from build123d import *

# Parameters (mm, degrees)
SKETCH_1_W               = 56
SKETCH_1_H               = 40
EXTRUDE_1_DEPTH          = 20
SKETCH_2_R               = 7.5
CUT_EXTRUDE_1_DEPTH      = 48
CUT_EXTRUDE_2_DEPTH      = 70.503098378
CUT_EXTRUDE_2_DEPTH_BACK = 48
SKETCH_5_R               = 4.15
CUT_EXTRUDE_3_DEPTH      = 10
SKETCH_6_R               = 2.1
CUT_EXTRUDE_4_DEPTH      = 57.255246128
CUT_EXTRUDE_5_DEPTH      = 10


with BuildPart() as part:
    # Эскиз1 → Бобышка-Вытянуть1 (new body)
    with BuildSketch(Plane(origin=(0, 0, 0), x_dir=(1, 0, 0), z_dir=(0, 1, 0))):
        with Locations((-4.217573352, -21.553347449)):
            Rectangle(SKETCH_1_W, SKETCH_1_H)
    extrude(amount=EXTRUDE_1_DEPTH)

    # Эскиз2 → Вырез-Вытянуть1 (cut)
    with BuildSketch(Plane.ZY.offset(28.217573352)):
        with Locations((39.13573239, 10)):
            Circle(SKETCH_2_R)
    extrude(amount=-CUT_EXTRUDE_1_DEPTH, mode=Mode.SUBTRACT)

    # Эскиз4 → Вырез-Вытянуть2 (cut, two sides: drawn at the far end of the back side and taken through both)
    with BuildSketch(Plane.ZY.offset(-19.782426648).offset(-CUT_EXTRUDE_2_DEPTH_BACK)):
        with BuildLine():
            Line((37.693734465, 13.535), (41.553347449, 13.535))
            Line((41.553347449, 13.535), (41.553347449, 6.465))
            Line((41.553347449, 6.465), (37.693734465, 6.465))
            ThreePointArc((37.693734465, 6.465), (34.158734465, 10), (37.693734465, 13.535))
        make_face()
    extrude(amount=CUT_EXTRUDE_2_DEPTH + CUT_EXTRUDE_2_DEPTH_BACK, mode=Mode.SUBTRACT)

    # Эскиз5 → Вырез-Вытянуть3 (cut)
    with BuildSketch(Plane(origin=(0, 0, 1.553347449), x_dir=(-1, 0, 0), z_dir=(0, 0, -1))):
        with Locations((-16.782426648, 10)):
            Circle(SKETCH_5_R)
        with Locations((25.217573352, 10)):
            Circle(SKETCH_5_R)
    extrude(amount=-CUT_EXTRUDE_3_DEPTH, mode=Mode.SUBTRACT)

    # Эскиз6 → Вырез-Вытянуть4 (cut, through all)
    with BuildSketch(Plane(origin=(0, 20, 0), x_dir=(1, 0, 0), z_dir=(0, 1, 0))):
        with Locations(Location((-25.217573352, -21.553347449, 0), (0, 0, 270))):
            Circle(SKETCH_6_R)
        with Locations(Location((16.782426648, -21.553347449, 0), (0, 0, 270))):
            Circle(SKETCH_6_R)
    extrude(amount=-CUT_EXTRUDE_4_DEPTH, mode=Mode.SUBTRACT)

    # Эскиз7 → Вырез-Вытянуть5 (cut)
    with BuildSketch(Plane.XZ):
        Polygon((-21.176121468, 21.553347449), (-23.19684741, 25.053347449), (-27.238299295, 25.053347449), (-29.259025237, 21.553347449), (-27.238299295, 18.053347449), (-23.19684741, 18.053347449), align=None)
        Polygon((20.823878532, 21.553347449), (18.80315259, 25.053347449), (14.761700705, 25.053347449), (12.740974763, 21.553347449), (14.761700705, 18.053347449), (18.80315259, 18.053347449), align=None)
    extrude(amount=-CUT_EXTRUDE_5_DEPTH, mode=Mode.SUBTRACT)


solid = part.part
Work out the finished part from the listing and answer in its coordinate system (mm). A direction names the side the tool comes from. Round coordinates to 2 decimals unless told otherwise and drop trailing zeros. Write each loop counter-clockwise with the first axis right and the second up, starting at its lowest first coordinate (ties: lowest second). Pieces come first, ordered by that corner, then holes.
1) Given pin 1 Ø1.2 at (x, z) = (21, 38.5) entering from -Y; pin 2 Ø2 at (x, z) = (-27, 20) entering from -Y; pin 3 Ø8 at (x, y) = (1, 12.5) entering from +Z; pin 4 Ø4 at (x, y) = (15.5, 10.5) entering from -Z, each flat-ended and moving along its own axis, determine where each tip first touches the part or whether it passes through.
2) A tool of negligible diameter and unlimited length cuts with its end or side. For faces 4 (the cylindrical face through (-4.55, 10.2, 31.64)), 5 (the flat face through (13.765, 4.93, 23.328)), 6 (the flat face through (-30, 6.465, 40)), from which of +Z, -Z, +X, -X, +Y, -Y can it reach the whole face along a straight path? Write none if from no direction.
3) Straight lines are drawn through the part: line 1 (X direction, y = 8.5, z = 6); line 2 (Y direction, x = -19, z = 38); line 3 (Y direction, x = 8, z = 35.5). For each, find the intervals that lie inside material, in ascending order.
4) The mould has two halves that part along Z. Classify faces 1 (the flat face through (22, 6.465, 40)), 2 (the flat face through (19.8, 4.93, 19.78)), 3 (the cylindrical face through (-30.19, 9.92, 34.16)): pulls with the +Z half, pulls with the -Z half, needs draft (parallel to the pull), parting line crosses it, or undercut.
5) A cutting plane is placed at B-B (x = -24). Give the vertices of the cut face in (y, z), plus the area to 3 significant figures.
6) A cutting plane is placed at C-C (x = 4). Give the vertices of the cut face in (y, z).
7) A cutting plane is placed at A-A (z = 8). Give the vertices of the cut face in (x, y).
Completed:
1. pin 1: stops at y = 0
1. pin 2: stops at y = 10
1. pin 3: stops at z = 35.39
1. pin 4: stops at z = 11.55
2. face 4: none
2. face 5: -Y
2. face 6: +Z, +X, -X
3. line 1: x = -32.22 to -29.09, -21.35 to 12.91, 20.65 to 23.78
3. line 2: y = 0 to 2.59, 17.41 to 20
3. line 3: y = 0 to 3.44, 16.56 to 20
4. face 1: needs draft
4. face 2: undercut
4. face 3: pulls with the +Z half
5. outline: (0, 1.55) - (6.03, 1.55) - (6.03, 11.55) - (13.97, 11.55) - (13.97, 1.55) - (20, 1.55) - (20, 19.84) - (10, 19.84) - (10, 18.05) - (0, 18.05) - close; (0, 25.05) - (10, 25.05) - (10, 23.26) - (20, 23.26) - (20, 41.55) - (17.1, 41.55) arc R7.5 cw (long way) to (2.9, 41.55) - (0, 41.55) - close
5. area: 492 mm2
6. outline: (0, 1.55) - (20, 1.55) - (20, 41.55) - (17.1, 41.55) arc R7.5 cw (long way) to (2.9, 41.55) - (0, 41.55) - close
7. outline: (-32.22, 0) - (23.78, 0) - (23.78, 20) - (-32.22, 20) - close; hole circle Ø8.3 at (-25.22, 10); hole circle Ø8.3 at (16.78, 10)
